Source: three-view drawing plus pictorial views. Frame: mm from the lowest corner of the part. A direction names the side the tool comes from. Give positions to 0.01 mm unless a question says otherwise; leave off trailing zeros. Order: outer loops, then holes, each group sorted by start corner. A loop starts at its lowest first (then second) coordinate and runs counter-clockwise, first axis right, second up. Notation, with made-up numbers: M 77.25,-10 L 119.25,-10 A7 ccw 119.25,2 Z; hole C 53.25,7.5 d6. An arc over 180 degrees is marked long. Use CSV: the item, a comma, the result in double quotes.
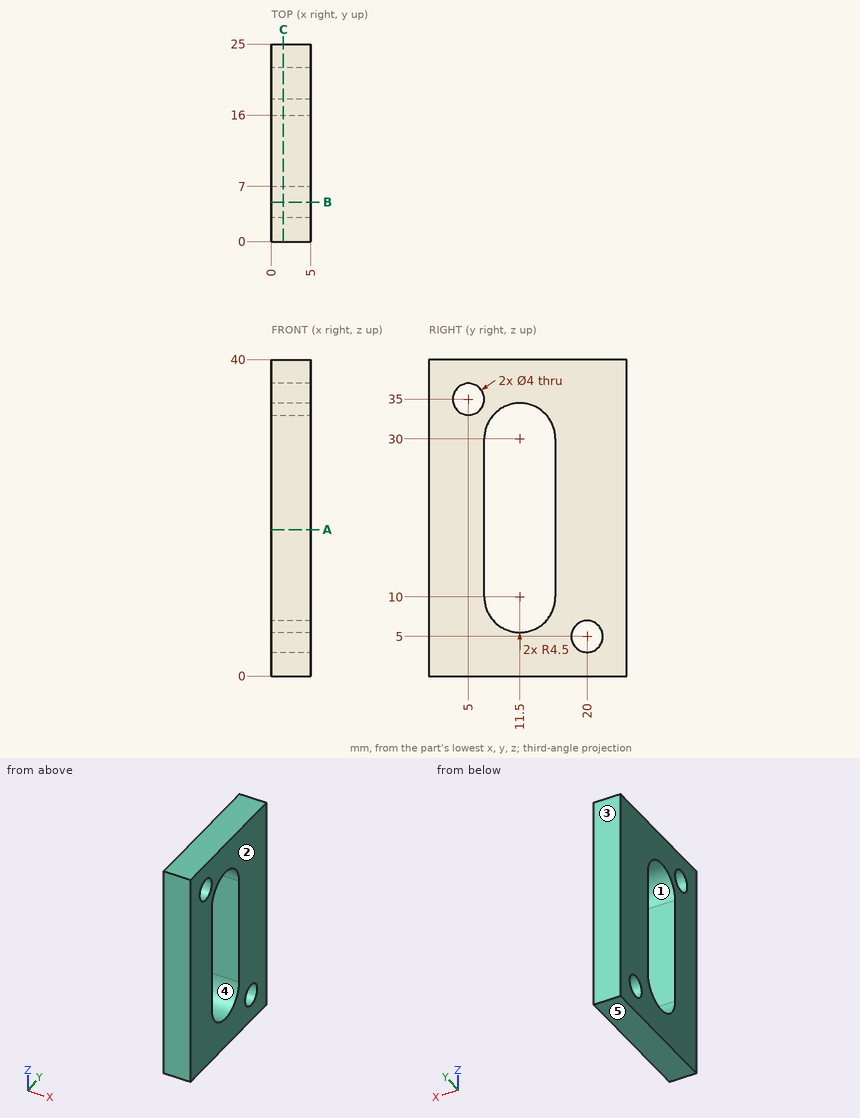
1. Line query: line 1 (Y direction, x = 1.9, z = 5); line 2 (Y direction, x = 3.5, z = 35); line 3 (Y direction, x = 3.05, z = 33.5). Output: solid intervals per line, ascending.
Answer:
line 1,"0 to 18, 22 to 25"
line 2,"0 to 3, 7 to 25"
line 3,"0 to 3.68, 6.32 to 8.67, 14.33 to 25"
2. Pull-direction query (Z, two-part tool) for the marked faces 3, 4 and 5; classes: +Z half, -Z half, draft (parallel to the pull), parting line (faces both ways), or undercut.
Answer:
face 3,"draft"
face 4,"undercut"
face 5,"-Z half"
3. Section A-A, the plane z = 18.5. Return the cut outline in (x, y).
Answer:
outline,"M 0,0 L 5,0 L 5,7 L 0,7 Z; M 0,16 L 5,16 L 5,25 L 0,25 Z"
4. Pin query (flat end, axial travel): pin 1 Ø3.5 at (y, z) = (20, 5) entering from +X. Return the tip coordinate at first contact, or that it passes through.
Answer:
pin 1,"through"
5. Section B-B, the plane y = 5. Return the cut outline in (x, z), plus the area to 3 significant figures.
Answer:
outline,"M 0,0 L 5,0 L 5,33 L 0,33 Z; M 0,37 L 5,37 L 5,40 L 0,40 Z"
area,"180 mm2"
6. Section C-C, the plane x = 1.5. Return the cut outline in (y, z), plus the area to 3 significant figures.
Answer:
outline,"M 0,0 L 25,0 L 25,40 L 0,40 Z; hole C 5,35 d4; hole M 7,10 A4.5 ccw 16,10 L 16,30 A4.5 ccw 7,30 Z; hole C 20,5 d4"
area,"731 mm2"
7. Reachability of the marked faces 1 and 2 from +Z, -Z, +X, -X, +Y, -Y: full face, straight path, thin tool, end or side. Return the list, or none.
Answer:
face 1,"+X, -X"
face 2,"+Z, -Z, +X, +Y, -Y"
